from build123d import *

# Parameters (mm, degrees)
F0_W           = 304.8
F0_H           = 38.1
F1_DEPTH       = 25.4
F2_D           = 7.9375
F2_CSINK_D     = 15.9004
F2_CSINK_ANGLE = 90
F4_D           = 6.35
F4_DEPTH       = 12.954
F4_TIP         = 1.9077324654


with BuildPart() as f1:
    # F0 (on Top) → F1 (new body)
    with BuildSketch(Plane.XY):
        with Locations((152.4, 19.05)):
            Rectangle(F0_W, F0_H)
    extrude(amount=F1_DEPTH)

    # F2 (through all)
    with Locations(Plane(origin=(0, 0, 0), x_dir=(1, 0, 0), z_dir=(0, 0, -1))):
        with Locations((50.8, -19.05), (101.6, -19.05), (152.4, -19.05), (203.2, -19.05), (254, -19.05)):
            CounterSinkHole(F2_D / 2, F2_CSINK_D / 2, counter_sink_angle=F2_CSINK_ANGLE)

    # F4
    with Locations(Plane.XZ):
        with Locations((25.4, 12.7), (127, 12.7), (177.8, 12.7), (279.4, 12.7)):
            Hole(F4_D / 2, depth=F4_DEPTH)
            with Locations((0, 0, -(F4_DEPTH + F4_TIP / 2))):  # 118° drill point
                Cone(0, F4_D / 2, F4_TIP, mode=Mode.SUBTRACT)


solid = f1.part
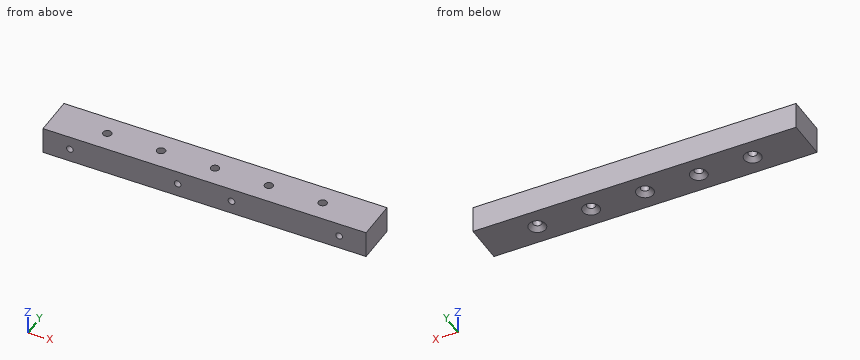
Verification items for the finished model (mm, model axes). Give positions to 0.01 mm unless a question says otherwise; leave off trailing zeros. Order: outer loops, then holes, each group sorted by start corner. A loop starts at its lowest first (then second) coordinate and runs counter-clockwise, first axis right, second up. Notation, with made-up numbers: M 44.25,0 L 55.25,0 A20 cw 55.25,4 Z; hole C 49,65 d11. An arc over 180 degrees is marked long. Answer as a JSON object with one key per item and string values. Group by question number.
1) Scan lines: line 1 along X through (y, z) = (10, 12.7) (3 decimals); line 2 along X through (y, z) = (19.05, 17); line 3 along Y through (x, z) = (153, 9.5). Record each from-to range of solid material in increasing order. Write a range as [from, to].
2) Cross-section at A-A (x = 152.4). Enter the section's corners in (y, z).
3) Depth check by flat-ended pin: pin 1 Ø10.5 at (x, y) = (101.6, 19.05) entering from -Z. Enter the tip coordinate at first touch or a pass-through.
4) Cross-section at B-B (y = 19.05). Give the number of separate pieces and of enclosed holes in the cut face, then the cut area to 3 significant figures.
5) Cross-section at C-C (y = 5.5). Enter the section's corners in (x, z) (3 decimals), then the cut area to 3 significant figures.
Result sheet:
{
 "1": {"line 1": "x = [0, 22.225], [28.575, 123.825], [130.175, 174.625], [180.975, 276.225], [282.575, 304.8]", "line 2": "x = [0, 46.83], [54.77, 97.63], [105.57, 148.43], [156.37, 199.23], [207.17, 250.03], [257.97, 304.8]", "line 3": "y = [0, 15.13], [22.97, 38.1]"},
 "2": {"outline": "M 0,0 L 11.1,0 L 15.08,3.98 L 15.08,25.4 L 0,25.4 Z; M 23.02,3.98 L 27,0 L 38.1,0 L 38.1,25.4 L 23.02,25.4 Z"},
 "3": {"pin 1": "stops at z = 2.7"},
 "4": {"separate pieces": "6", "enclosed holes": "0", "area": "6,650 mm2"},
 "5": {"outline": "M 0,0 L 304.8,0 L 304.8,25.4 L 0,25.4 Z; hole C 25.4,12.7 d6.35; hole C 127,12.7 d6.35; hole C 177.8,12.7 d6.35; hole C 279.4,12.7 d6.35", "area": "7,620 mm2"}
}
